Work out the finished part from the listing and answer in its coordinate system (mm). A direction names the side the tool comes from. Give positions to 0.01 mm unless a question says otherwise; leave off trailing zeros. Order: outer loops, then holes, each group sorted by start corner. A loop starts at its lowest first (then second) coordinate and runs counter-clockwise, first axis right, second up. Notation, with made-up numbers: (-16.5, 0) -> (2.5, 0) arc R4 ccw to (2.5, 7) -> close; hole circle Ø8 at (48, -31). An arc over 180 degrees is marked (long way). Use a Markdown table: item, result. Add a question column.
```python
from build123d import *

# Parameters (mm, degrees)
F1_DEPTH = 72.898
F2_W     = 24.1890717298
F2_H     = 18.2968638837
F3_DEPTH = 12.7


# Not quite as in the source:
# - a length typed as a fraction of an inch, garbled in the dataset ("3 / 203.2 mm" for 3/8 in), is restored


with BuildPart() as f1:
    # F0 (on Right) → F1 (new body)
    with BuildSketch(Plane.YZ):
        Polygon((-3.8764555939, 0), (0, 0), (6.0472693294, 0), (6.0472693294, 16.9013366103), (-15.3507553041, 16.9013366103), (-15.3507553041, 50.3938943148), (-33.6476191878, 50.3938943148), (-33.6476191878, 0), align=None)
    extrude(amount=F1_DEPTH)

    # F2 (on face) → F3 (cut)
    with BuildSketch(Plane.XY.offset(50.3938943148)):
        with Locations((38.2993584499, -24.499187246)):
            Rectangle(F2_W, F2_H)
    extrude(amount=-F3_DEPTH, mode=Mode.SUBTRACT)


solid = f1.part
```
1) Determine the mould class of faces 4 (the flat face through (36, -33.648, 26)), 5 (the flat face through (72.898, -18, 20)), 6 (the flat face through (38, -24, 37.694)) for opening direction X: released by +X, released by -X, zero draft, split by the parting line, or undercut.
2) The part is cut by section C-C, the plane z = 32. Determine the outline of the cut face in (x, y).
3) Straight lines are drawn through the part: line 1 (Z direction, x = 7, y = -15); line 2 (Y direction, x = 3, z = 31.5); line 3 (Z direction, x = 30, y = -18.5). For each, find the intervals that lie inside material, in ascending order.
4) Flat-ended cylindrical pins translate along their axes: pin 1 (9 mm diameter, centred on x = 44.5, y = -21.5, fed in from +Z); pin 2 (4 mm diameter, centred on x = 27.5, z = 24, fed in from +Y). Find the tip coordinate at first contact, or state that the pin passes through.
5) The part is cut by section D-D, the plane x = 66. Determine the outline of the cut face in (y, z), then the cut area to 3 significant figures.
6) The part is cut by section A-A, the plane x = 31. Determine the outline of the cut face in (y, z), then the cut area to 3 significant figures.
7) Which of the six approach directions +Z, -Z, +X, -X, +Y, -Y give full straight-line access (tool end or side, diameter ignored) to faces 1 (the flat face through (36, 6.047, 8)), 2 (the flat face through (36, -15.351, 33)), 3 (the flat face through (50.394, -25, 44))?
8) The part is cut by section B-B, the plane y = -26. Determine the outline of the cut face in (x, z).
A:
| question | item | result |
|---|---|---|
| 1 | face 4 | zero draft |
| 1 | face 5 | released by +X |
| 1 | face 6 | undercut |
| 2 | outline | (0, -33.65) -> (72.9, -33.65) -> (72.9, -15.35) -> (0, -15.35) -> close |
| 3 | line 1 | 0 to 16.9 |
| 3 | line 2 | -33.65 to -15.35 |
| 3 | line 3 | 0 to 37.69 |
| 4 | pin 1 | z = 37.69 |
| 4 | pin 2 | y = -15.35 |
| 5 | outline | (-33.65, 0) -> (6.05, 0) -> (6.05, 16.9) -> (-15.35, 16.9) -> (-15.35, 50.39) -> (-33.65, 50.39) -> close |
| 5 | area | 1,280 mm^2 |
| 6 | outline | (-33.65, 0) -> (6.05, 0) -> (6.05, 16.9) -> (-15.35, 16.9) -> (-15.35, 37.69) -> (-33.65, 37.69) -> close |
| 6 | area | 1,050 mm^2 |
| 7 | face 1 | +Z, -Z, +X, -X, +Y |
| 7 | face 2 | +Z, +X, -X, +Y |
| 7 | face 3 | +Z, +Y, -Y |
| 8 | outline | (0, 0) -> (72.9, 0) -> (72.9, 50.39) -> (50.39, 50.39) -> (50.39, 37.69) -> (26.2, 37.69) -> (26.2, 50.39) -> (0, 50.39) -> close |
